Could you check a few things on this drawing? It's one solid part, dimensions in mm from its lowest x, y, z. A direction names the side the tool comes from. Give positions to 0.01 mm unless a question says otherwise; leave off trailing zeros. Loops run counter-clockwise (first coordinate to the right, second up) from the corner with the lowest first, then second, coordinate; pieces in that order, holes last.
Q1. I need wall thicknesses on probe 1 along Y at (x, z) = (27, 13.75); probe 2 along Z at (x, y) = (5.5, 38); probe 3 along Y at (x, z) = (22.5, 20.25). Which ranges of each line are inside material? Lowest first, please.
Q2. Suppose I cut it at B-B (y = 33). List the corners of the cut face in (x, z) for me, and give its area (3 significant figures).
Q3. For the marked faces 1 and 2, which set-ups out of +Z, -Z, +X, -X, +Y, -Y let a thin tool reach every point of the face, with its end or its side?
Q4. I'm going to push flat-ended pins straight in: P1, Ø11, axis at x = 16.5, z = 9.5, coming from the +Y side; P2, Ø3, axis at x = 39.5, y = 32, coming from the -Z side. Where does each tip first touch, or does it pass through?
Q5. Suppose I cut it at A-A (x = 22.5). List the corners of the cut face in (y, z) for me.
Q6. Suppose I cut it at D-D (z = 12). List the corners of the cut face in (x, y) for me, and give its area (3 significant figures).
Q7. Suppose I cut it at C-C (x = 37). List the corners of the cut face in (y, z) for me.
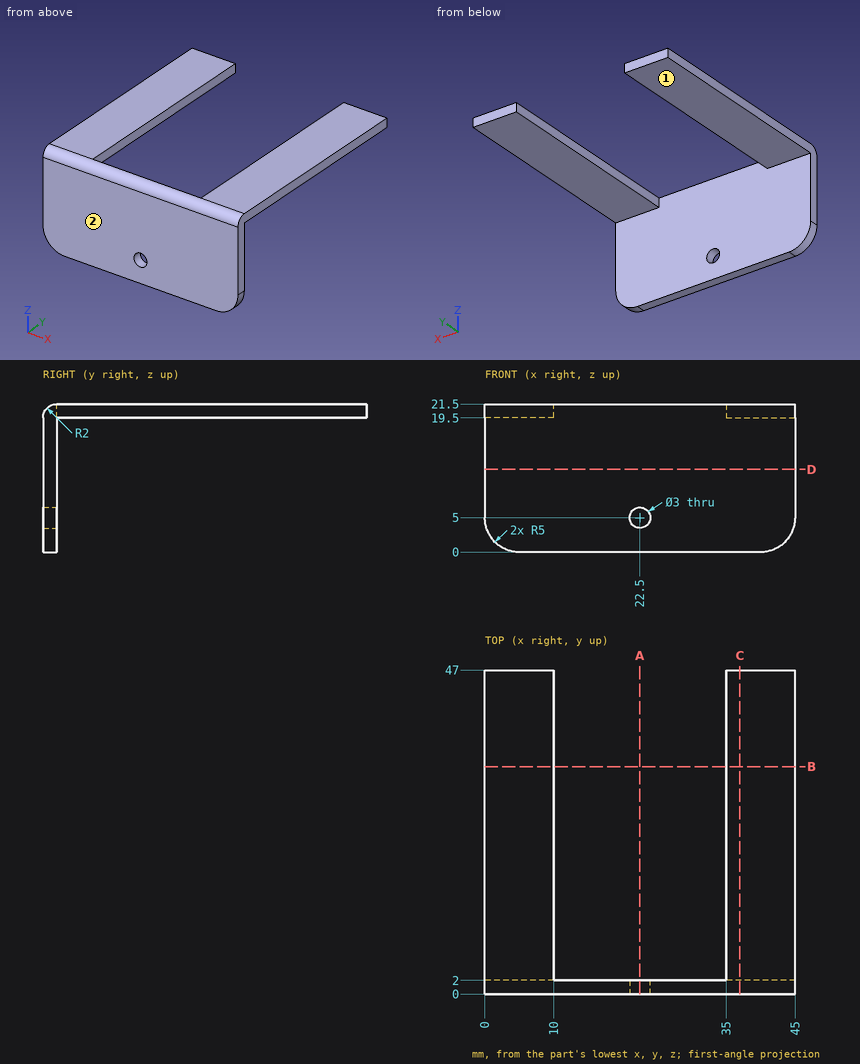
Solutions:
1. probe 1: y = 0 to 2
1. probe 2: z = 19.5 to 21.5
1. probe 3: y = 0.15 to 2
2. outline: (0, 19.5) - (10, 19.5) - (10, 21.5) - (0, 21.5) - close; (35, 19.5) - (45, 19.5) - (45, 21.5) - (35, 21.5) - close
2. area: 40.0 mm2
3. face 1: -Z, +X, -X, +Y
3. face 2: +Z, -Z, +X, -X, -Y
4. P1: stops at y = 2
4. P2: stops at z = 19.5
5. outline: (0, 0) - (2, 0) - (2, 3.5) - (0, 3.5) - close; (0, 6.5) - (2, 6.5) - (2, 21.5) arc R2 ccw to (0, 19.5) - close
6. outline: (0, 0) - (45, 0) - (45, 2) - (0, 2) - close
6. area: 90.0 mm2
7. outline: (0, 0) - (2, 0) - (2, 19.5) - (47, 19.5) - (47, 21.5) - (2, 21.5) arc R2 ccw to (0, 19.5) - close
